Design review of the part built by this model. Coordinates are the model's own, in mm. A direction names the side the tool comes from. Give positions to 0.01 mm unless a question says otherwise; leave off trailing zeros. Order: outer loops, then holes, each group sorted by start corner. A loop starts at its lowest first (then second) coordinate and runs counter-clockwise, first axis right, second up. Notation, with made-up numbers: (-10.75, 55.25) -> (-1.75, 55.25) arc R13 ccw to (-1.75, 67.25) -> close; hole circle Ø4 at (71, 11). An arc over 180 degrees is marked (long way). Return JSON: item names as keys, results as strings.
```python
from build123d import *

# Parameters (mm, degrees)
SKETCH_1_W          = 15
SKETCH_1_H          = 15
SKETCH_1_W_2        = 13
SKETCH_1_H_2        = 13
EXTRUDE_1_DEPTH     = 460
SKETCH_2_R          = 1.45
CUT_EXTRUDE_1_DEPTH = 461.305605006
SKETCH_3_R          = 1.45
CUT_EXTRUDE_2_DEPTH = 461.305605006


with BuildPart() as part:
    # 草图1 → 拉伸-薄壁1 (new body)
    with BuildSketch(Plane(origin=(0, 0, 0), x_dir=(1, 0, 0), z_dir=(0, 1, 0))):
        Rectangle(SKETCH_1_W, SKETCH_1_H)
        Rectangle(SKETCH_1_W_2, SKETCH_1_H_2, mode=Mode.SUBTRACT)
    extrude(amount=EXTRUDE_1_DEPTH)

    # 草图2 → 切除-拉伸1 (cut, through all)
    with BuildSketch(Plane.XY.offset(7.5)):
        with Locations((0, 7.5)):
            Circle(SKETCH_2_R)
        with Locations((0, 27.5)):
            Circle(SKETCH_2_R)
        with Locations(Location((0, 432.5, 0), (0, 0, 180))):
            Circle(SKETCH_2_R)
        with Locations(Location((0, 452.5, 0), (0, 0, 180))):
            Circle(SKETCH_2_R)
        with Locations((0, 80)):
            Circle(SKETCH_2_R)
        with Locations((0, 100)):
            Circle(SKETCH_2_R)
        with Locations((0, 350)):
            Circle(SKETCH_2_R)
        with Locations((0, 370)):
            Circle(SKETCH_2_R)
        with Locations((0, 330)):
            Circle(SKETCH_2_R)
        with Locations((0, 230)):
            Circle(SKETCH_2_R)
        with Locations((0, 255)):
            Circle(SKETCH_2_R)
        with Locations((0, 280)):
            Circle(SKETCH_2_R)
        with Locations((0, 205)):
            Circle(SKETCH_2_R)
        with Locations((0, 180)):
            Circle(SKETCH_2_R)
    extrude(amount=-CUT_EXTRUDE_1_DEPTH, mode=Mode.SUBTRACT)

    # 草图3 → 切除-拉伸2 (cut, through all)
    with BuildSketch(Plane(origin=(7.5, 0, 0), x_dir=(0, 0, -1), z_dir=(1, 0, 0))):
        with Locations((0, 15)):
            Circle(SKETCH_3_R)
        with Locations((0, 35)):
            Circle(SKETCH_3_R)
        with Locations((0, 425)):
            Circle(SKETCH_3_R)
        with Locations((0, 445)):
            Circle(SKETCH_3_R)
        with Locations((0, 172.5)):
            Circle(SKETCH_3_R)
        with Locations((0, 192.5)):
            Circle(SKETCH_3_R)
        with Locations((0, 152.5)):
            Circle(SKETCH_3_R)
        with Locations((0, 307.5)):
            Circle(SKETCH_3_R)
        with Locations((0, 267.5)):
            Circle(SKETCH_3_R)
        with Locations((0, 287.5)):
            Circle(SKETCH_3_R)
        with Locations((0, 55)):
            Circle(SKETCH_3_R)
        with Locations((0, 405)):
            Circle(SKETCH_3_R)
    extrude(amount=-CUT_EXTRUDE_2_DEPTH, mode=Mode.SUBTRACT)


solid = part.part
```
Item 1: Add section A-A (y = 391). Give the boundary of the cut face in (x, z), plus the area to 3 significant figures.
Result set:
{"outline": "(-7.5, -7.5) -> (7.5, -7.5) -> (7.5, 7.5) -> (-7.5, 7.5) -> close; hole (-6.5, -6.5) -> (6.5, -6.5) -> (6.5, 6.5) -> (-6.5, 6.5) -> close", "area": "56.0 mm^2"}
Item 2: Mouldability with a two-part tool opening along Z and no side actions: class faces 1 (the face through (-7, 0, 0)), 2 (the face through (0, 227, 7.5)), 3 (the face through (-6.5, 227, 0)) as released by +Z, released by -Z, zero draft, split by the parting line, or undercut.
Result set:
{"face 1": "zero draft", "face 2": "released by +Z", "face 3": "undercut"}
Item 3: Wall thickness on L1, parallel to X at y = 350, z = -7; L2, parallel to X at y = 210, z = 5.25: over which ranges is each line inside the solid? List them lowest first. Write a range as [from, to].
Result set:
{"L1": "x = [-7.5, -1.45], [1.45, 7.5]", "L2": "x = [-7.5, -6.5], [6.5, 7.5]"}
Item 4: Machinability: for faces 4 (the face through (6.5, 227, 0)), 5 (the face through (-7.5, 227, 0)), which of the approach directions +Z, -Z, +X, -X, +Y, -Y give a long, thin tool a straight path to every point of the face, cutting with its end or side? Answer none if there is none.
Result set:
{"face 4": "+Y, -Y", "face 5": "+Z, -Z, -X, +Y, -Y"}
